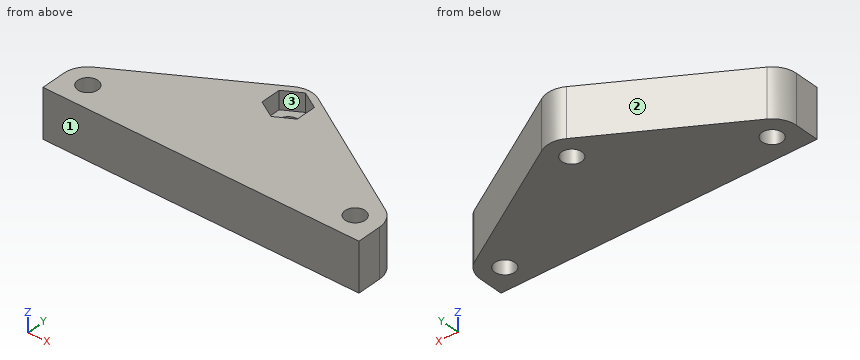
```python
from build123d import *

# Parameters (mm, degrees)
SKETCH1_R           = 1.65
BOSS_EXTRUDE1_DEPTH = 8
CUT_EXTRUDE1_DEPTH  = 3


with BuildPart() as part:
    # Sketch1 → Boss-Extrude1 (new body)
    with BuildSketch(Plane.XY):
        with BuildLine():
            Line((0, 0), (52, 0))
            Line((52, 0), (52, 4))
            ThreePointArc((52, 4), (51.538809184, 5.864625849), (50.261585222, 7.29927754))
            Line((50.261585222, 7.29927754), (28.036121371, 20.442994302))
            ThreePointArc((28.036121371, 20.442994302), (26.00069939, 20.999999939), (23.965082751, 20.443706113))
            Line((23.965082751, 20.443706113), (1.965082751, 7.443706113))
            ThreePointArc((1.965082751, 7.443706113), (0.525833266, 5.982464502), (0, 4))
            Line((0, 4), (0, 0))
        make_face()
        with Locations((26, 17)):
            Circle(SKETCH1_R, mode=Mode.SUBTRACT)
        with Locations((4, 4)):
            Circle(SKETCH1_R, mode=Mode.SUBTRACT)
        with Locations((48, 4)):
            Circle(SKETCH1_R, mode=Mode.SUBTRACT)
    extrude(amount=BOSS_EXTRUDE1_DEPTH)

    # Sketch2 → Cut-Extrude1 (cut)
    with BuildSketch(Plane.XY.offset(8)):
        Polygon((26, 13.651368439), (28.9, 15.325684219), (28.9, 18.674315781), (26, 20.348631561), (23.1, 18.674315781), (23.1, 15.325684219), align=None)
    extrude(amount=-CUT_EXTRUDE1_DEPTH, mode=Mode.SUBTRACT)


solid = part.part
```
Geometry check sheet. Reference: the model listing, model coordinates, mm. Face numbers are marked on the shaded views. Coordinates: 2 decimals unless noted, no trailing zeros. Write each loop counter-clockwise with the first axis right and the second up, starting at its lowest first coordinate (ties: lowest second). Pieces come first, ordered by that corner, then holes. Notation, with made-up numbers: (19, 4.5) -> (31, 4.5) arc R17 ccw to (31, 33.5) -> close; hole circle Ø8 at (54.5, 83). An arc over 180 degrees is marked (long way). Use CSV: the item, a comma, the result in double quotes. Start each with the question number.
Item 1: Thickness scan on line 1 (Y direction, x = 26, z = 3.4); line 2 (X direction, y = 5, z = 3.75); line 3 (Y direction, x = 49, z = 1.75). Record the ranges inside material, lowest first.
Item 2: Cross-section at C-C, the plane y = 16. Record the cut outline in (x, z).
Item 3: Cross-section at B-B, the plane x = 48. Record the cut outline in (y, z).
Item 4: Cross-section at D-D, the plane z = 2. Record the cut outline in (x, y).
Item 5: Cross-section at A-A, the plane z = 6.5. Record the cut outline in (x, y), plus the area to 3 significant figures.
Item 6: Depth check by flat-ended pin: pin 1 Ø4 at (x, z) = (38.5, 6.5) entering from +Y; pin 2 Ø1 at (y, z) = (5, 6.5) entering from -X; pin 3 Ø2.5 at (y, z) = (17.5, 6) entering from -X; pin 4 Ø4 at (x, y) = (4, 4) entering from +Z. Enter the tip coordinate at first touch or a pass-through.
Item 7: Mould release check, pull along Y, two halves, no side actions. Record for the marked faces 1, 2 and 3: released by +Y, released by -Y, zero draft, split by the parting line, or undercut.
Answers:
1,line 1,"0 to 15.35, 18.65 to 21"
1,line 2,"0.13 to 2.69, 5.31 to 46.69, 49.31 to 51.87"
1,line 3,"0 to 2.69, 5.31 to 8.05"
2,outline,"(16.44, 0) -> (24.69, 0) -> (24.69, 5) -> (23.1, 5) -> (23.1, 8) -> (16.44, 8) -> close; (27.31, 0) -> (35.55, 0) -> (35.55, 8) -> (28.9, 8) -> (28.9, 5) -> (27.31, 5) -> close"
3,outline,"(0, 0) -> (2.35, 0) -> (2.35, 8) -> (0, 8) -> close; (5.65, 0) -> (8.64, 0) -> (8.64, 8) -> (5.65, 8) -> close"
4,outline,"(0, 0) -> (52, 0) -> (52, 4) arc R4 ccw to (50.26, 7.3) -> (28.04, 20.44) arc R4 ccw to (23.97, 20.44) -> (1.97, 7.44) arc R4 ccw to (0, 4) -> close; hole circle Ø3.3 at (4, 4); hole circle Ø3.3 at (26, 17); hole circle Ø3.3 at (48, 4)"
5,outline,"(0, 0) -> (52, 0) -> (52, 4) arc R4 ccw to (50.26, 7.3) -> (28.04, 20.44) arc R4 ccw to (23.97, 20.44) -> (1.97, 7.44) arc R4 ccw to (0, 4) -> close; hole circle Ø3.3 at (4, 4); hole (23.1, 15.33) -> (26, 13.65) -> (28.9, 15.33) -> (28.9, 18.67) -> (26, 20.35) -> (23.1, 18.67) -> close; hole circle Ø3.3 at (48, 4)"
5,area,"677 mm^2"
6,pin 1,"y = 15.44"
6,pin 2,"x = 0.03"
6,pin 3,"x = 16.87"
6,pin 4,"z = 8"
7,face 1,"released by -Y"
7,face 2,"released by +Y"
7,face 3,"undercut"
